```python
from build123d import *

# Parameters (mm, degrees)
F0_R     = 1.27
F1_DEPTH = 12.7


# Not quite as in the source:
# - a feature names something its author has since deleted; it is built from what else it names


with BuildPart() as f1:
    # F0 (on Front) → F1 (new body)
    with BuildSketch(Plane.XZ):
        Polygon((2.54, -3.81), (0, 0), (-5.08, 0), (-7.62, 0), (-10.16, 0), (-10.16, -1.27), (-7.62, -3.81), (-2.54, -3.81), (1.605475081, -12.7), (4.145475081, -12.7), align=None)
        with Locations((-2.54, -1.905)):
            Circle(F0_R, mode=Mode.SUBTRACT)
        Polygon((-7.62, 0), (-5.08, 0), (-5.08, 3.175), align=None)
    extrude(amount=F1_DEPTH)


solid = f1.part
```
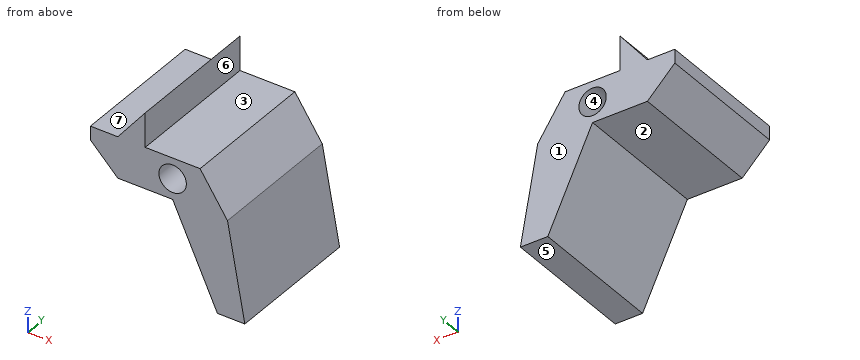
For this review, take the finished solid that the model builds, in its own axes (mm). Face numbers are marked on the shaded views. A direction names the side the tool comes from. Give positions to 0.01 mm unless a question says otherwise; leave off trailing zeros. Loops run counter-clockwise (first coordinate to the right, second up) from the corner with the lowest first, then second, coordinate; pieces in that order, holes last. Notation, with made-up numbers: M 15.25,-23 L 63.25,-23 A22 ccw 63.25,1 Z; hole C -37.75,66 d3. An arc over 180 degrees is marked long. One line per item, written item: value. Start each with the question number.
Q1. Draft analysis for pull direction Z (two halves, no side actions). For the marked faces 4, 5, 6 and 7, state which applies: released by +Z, released by -Z, zero draft, split by the parting line, or undercut.
Q2. Add section C-C (z = -9.5). Give the boundary of the cut face in (x, y), and give its area (3 significant figures).
Q3. Add section B-B (x = -8.5). Give the boundary of the cut face in (y, z), and give its area (3 significant figures).
Q4. Clearance check with flat-ended pins moving along their axes: pin 1 Ø1.3 at (x, y) = (-8.5, -7.5) entering from +Z; pin 2 Ø4 at (x, y) = (-6, -9) entering from -Z; pin 3 Ø1 at (y, z) = (-3, 1) entering from +X. State where each tip first meets the part, or that it passes through.
Q5. For L1, parallel to Z at x = -4.25, y = -7.25; L2, parallel to Z at x = -3.5, y = -7.5; L3, parallel to Z at x = -3.25, y = -9, list the stretches that pass through material, from the lowest coordinate up.
Q6. Machinability: for the marked faces 1, 2 and 3, which of the approach directions +Z, -Z, +X, -X, +Y, -Y give a long, thin tool a straight path to every point of the face, cutting with its end or side? Answer none if there is none.
Q7. Add section A-A (y = -4). Give the boundary of the cut face in (x, z) (3 decimals), and give its area (3 significant figures).
Reply:
1. face 4: undercut
1. face 5: released by -Z
1. face 6: zero draft
1. face 7: released by +Z
2. outline: M 0.11,-12.7 L 3.57,-12.7 L 3.57,0 L 0.11,0 Z
2. area: 43.9 mm²
3. outline: M -12.7,-2.93 L 0,-2.93 L 0,0 L -12.7,0 Z
3. area: 37.2 mm²
4. pin 1: z = 0
4. pin 2: z = -3.81
4. pin 3: x = -5.08
5. L1: -3.81 to 0
5. L2: -3.81 to -2.74, -1.07 to 0
5. L3: -3.81 to -2.96, -0.85 to 0
6. face 1: +Z, -Z, +X, -X, +Y
6. face 2: -Z, -X, +Y, -Y
6. face 3: +Z, +X, +Y, -Y
7. outline: M -10.16,-1.27 L -7.62,-3.81 L -2.54,-3.81 L 1.605,-12.7 L 4.145,-12.7 L 2.54,-3.81 L 0,0 L -5.08,0 L -5.08,3.175 L -7.62,0 L -10.16,0 Z; hole C -2.54,-1.905 d2.54
7. area: 73.2 mm²
